For this review, take the finished solid that the model builds, in its own axes (mm). A direction names the side the tool comes from. Coordinates: 2 decimals unless noted, no trailing zeros. Loops run counter-clockwise (first coordinate to the right, second up) from the corner with the lowest first, then second, coordinate; pieces in that order, holes last. Notation, with made-up numbers: (16.25, 31.5) -> (62.25, 31.5) arc R30 cw to (62.25, 58.5) -> close; hole circle Ø2 at (-15, 48). An arc over 180 degrees is marked (long way). Use a Markdown table: item, result.
from build123d import *

# Parameters (mm, degrees)
F0_R      = 17.5
F0_R_2    = 15
F1_DEPTH  = 38.6
F1_TAPER  = -1.5
F2_R      = 22.25
F2_R_2    = 18.5107765726
F2_R_3    = 14
F3_DEPTH  = 2.8
F5_R      = 20.05
F5_R_2    = 17.55
F6_DEPTH  = 45
F6_TAPER  = -0.75
F7_SIZE   = 1.6109
F8_R      = 31.610490496
F9_DEPTH  = 38.6
F10_R     = 18.3
F10_R_2   = 15.8
F11_DEPTH = 38.6
F11_TAPER = -1.5


# Not quite as in the source:
# - a fillet or chamfer is up to 0.001 mm smaller than in the source, because OpenCascade refuses the exact size


with BuildPart() as f1:
    # F0 (on Top) → F1 (new body)
    with BuildSketch(Plane.XY):
        Circle(F0_R)
        Circle(F0_R_2, mode=Mode.SUBTRACT)
    extrude(amount=F1_DEPTH, taper=F1_TAPER)

    # F2 (on face) → F3 (join)
    with BuildSketch(Plane.XY.offset(38.6)):
        Circle(F2_R)
        Circle(F2_R_2, mode=Mode.SUBTRACT)
        Circle(F2_R_2)
        Circle(F2_R_3, mode=Mode.SUBTRACT)
    extrude(amount=F3_DEPTH)

    # F5 (on offset) → F6 (join, through all)
    with BuildSketch(Plane.XY.offset(86.4)):
        Circle(F5_R)
        Circle(F5_R_2, mode=Mode.SUBTRACT)
    extrude(amount=-F6_DEPTH, taper=F6_TAPER)

    # F7 (size 1.611 in the source; OpenCascade refuses exactly that, so slightly less here)
    f7_edges = [f1.edges().sort_by_distance(p)[0] for p in [
        (-22.25, 0, 41.4),
    ]]
    chamfer(f7_edges, length=F7_SIZE)

    # F8 (on Top) → F9 (cut, through all)
    with BuildSketch(Plane.XY):
        Circle(F8_R)
    extrude(amount=F9_DEPTH, mode=Mode.SUBTRACT)

    # F10 (on Top) → F11 (join, through all)
    with BuildSketch(Plane.XY):
        Circle(F10_R)
        Circle(F10_R_2, mode=Mode.SUBTRACT)
    extrude(amount=F11_DEPTH, taper=F11_TAPER)


solid = f1.part
(1) For faces 1 (the face through (-6, 13, 41.4)), 2 (the face through (-9, -11, 38.6)), 3 (the face through (-16.399, 15.038, 39.186)), list the 3-axis set-ups (+Z, -Z, +X, -X, +Y, -Y) from which the entire face can be reached by the end or side of a thin tool; tool diameter is ignored.
Found:
| item | result |
|---|---|
| face 1 | +Z |
| face 2 | -Z |
| face 3 | +Z, -Z |
(2) Take a section at B-B on z = 69.5. Write out the cut boundary in (x, y), plus the area to 3 significant figures.
Found:
| item | result |
|---|---|
| outline | circle Ø40.54 at (0, 0); hole circle Ø34.66 at (0, 0) |
| area | 348 mm^2 |
(3) Take a section at A-A on z = 49. Write out the cut boundary in (x, y), plus the area to 3 significant figures.
Found:
| item | result |
|---|---|
| outline | circle Ø41.08 at (0, 0); hole circle Ø34.12 at (0, 0) |
| area | 411 mm^2 |
(4) For pin 1 Ø1.5 at (y, z) = (16, 38) entering from -X; pin 2 Ø12 at (x, z) = (3.5, 39) entering from -Y; pin 3 Ø5 at (x, z) = (3, 50) entering from +Y, all flat-tipped, find the tip position at first contact; note any pin that passes through.
Found:
| item | result |
|---|---|
| pin 1 | stops at x = -15.91 |
| pin 2 | stops at y = -22.25 |
| pin 3 | stops at y = 20.53 |
(5) For line 1 along Y through (x, z) = (0, 39.6); line 2 along Z through (x, y) = (10.5, -9.5); line 3 along Y through (x, z) = (11.5, 36.5), list the stretches that pass through material, from the lowest coordinate up.
Found:
| item | result |
|---|---|
| line 1 | y = -22.25 to -14, 14 to 22.25 |
| line 2 | z = 38.6 to 41.4 |
| line 3 | y = -15.44 to -9.39, 9.39 to 15.44 |
(6) Mouldability with a two-part tool opening along Y and no side actions: class faces 4 (the face through (-4.411, -19.865, 63.585)), 5 (the face through (-3.74, 16.84, 63.59)), 6 (the face through (12.932, -5.362, 39.98)), 7 (the face through (-14, -8, 0)) as pulls with the +Y half, pulls with the -Y half, needs draft (parallel to the pull), parting line crosses it, or undercut.
Found:
| item | result |
|---|---|
| face 4 | parting line crosses it |
| face 5 | undercut |
| face 6 | undercut |
| face 7 | needs draft |
